from build123d import *
from build123d.topology import SkipClean

# Parameters (mm, degrees)
SKETCH7_W           = 80
SKETCH7_H           = 28
EXTRUDE2_DEPTH      = 4
SKETCH8_W           = 28
SKETCH8_H           = 20
EXTRUDE3_DEPTH      = 9.5
EXTRUDE6_DEPTH      = 28
SKETCH15_R          = 7.5
EXTRUDE7_DEPTH      = 25
SKETCH16_W          = 3
SKETCH16_H          = 3
SKETCH8_4_W         = 28
SKETCH8_4_H         = 20
EXTRUDE8_DEPTH      = 9.5
EXTRUDE9_DEPTH      = 28
SKETCH19_R          = 7.5
EXTRUDE10_DEPTH     = 25
SKETCH20_W          = 3
SKETCH20_H          = 3
FILLET1_R           = 2.5
EXTRUDE11_DEPTH     = 16
SKETCH23_R          = 4
EXTRUDE12_DEPTH     = 40
SKETCH25_W          = 28
SKETCH25_H          = 5
EXTRUDE13_DEPTH     = 12
EXTRUDE14_REACH     = 90.69
FILLET2_R           = 2.5
FILLET9_R           = 2
FILLET10_R          = 2
FILLET11_R          = 2
SKETCH27_W          = 28
SKETCH27_H          = 5
EXTRUDE15_DEPTH     = 12
EXTRUDE16_REACH     = 90.69
FILLET12_R          = 2
FILLET13_R          = 2
FILLET14_R          = 2
FILLET15_R          = 2
SKETCH30_W          = 3
SKETCH30_H          = 3
EXTRUDE17_DEPTH     = 12
SKETCH31_W          = 3
SKETCH31_H          = 3
EXTRUDE18_DEPTH     = 12
FILLET16_R          = 2
EXTRUDE19_OUTLINE_R = 1.5
EXTRUDE19_DEPTH     = 4


# Read off the part's stored shape, not the designer's step: Extrude19
with BuildPart() as part:
    # Sketch7 → Extrude2 (new body)
    with BuildSketch(Plane(origin=(0, 0, 0), x_dir=(1, 0, 0), z_dir=(0, 1, 0))):
        with Locations((0, 23)):
            Rectangle(SKETCH7_W, SKETCH7_H)
    extrude(amount=EXTRUDE2_DEPTH)


with BuildPart() as body_2:
    # Sketch8 → Extrude3 (new body)
    with BuildSketch(Plane(origin=(0, 4, 0), x_dir=(1, 0, 0), z_dir=(0, 1, 0))):
        with Locations((-23, 24)):
            Rectangle(SKETCH8_W, SKETCH8_H)
    extrude(amount=EXTRUDE3_DEPTH)

    # Sketch10 → Extrude6 (cut)
    with BuildSketch(Plane(origin=(-9, 0, 0), x_dir=(0, 0, -1), z_dir=(1, 0, 0))):
        with BuildLine():
            Line((31.5, 13.5), (24, 13.5))
            Line((24, 13.5), (16.5, 13.5))
            ThreePointArc((16.5, 13.5), (17.126403912, 10.499387259), (18.900980486, 8))
            Line((18.900980486, 8), (29.099019514, 8))
            ThreePointArc((29.099019514, 8), (30.873596088, 10.499387259), (31.5, 13.5))
        make_face()
    extrude(amount=-EXTRUDE6_DEPTH, mode=Mode.SUBTRACT)

    # Sketch15 → Extrude7 (cut)
    with SkipClean():  # the faces are left unmerged after this step: merging them gives an invalid solid
        with BuildSketch(Plane.ZY.offset(35.5)):
            with Locations((-24, 13.5)):
                Circle(SKETCH15_R)
        extrude(amount=-EXTRUDE7_DEPTH, mode=Mode.SUBTRACT)


with BuildPart() as cut_sweep1_tool:
    # Cut-Sweep1: sweep along a path in Sketch17
    with SkipClean():  # the faces are left unmerged after this step: merging them gives an invalid solid
        with BuildLine(Plane(origin=(-23, 0, 0), x_dir=(0, 0, -1), z_dir=(1, 0, 0))) as cut_sweep1_path:
            CenterArc((24, 13.5), 12.806248475, 0, 360)
        # Sketch16 → Cut-Sweep1 (sweep)
        with BuildSketch(Plane.XY.offset(-14)):
            with Locations((-23, 5.5)):
                Rectangle(SKETCH16_W, SKETCH16_H)
        sweep(path=cut_sweep1_path.line)


with BuildPart() as part_1:
    with SkipClean():  # the faces are left unmerged after this step: merging them gives an invalid solid
        add(part.part)

        # Cut-Sweep1: cut by cut_sweep1_tool
        add(cut_sweep1_tool.part, mode=Mode.SUBTRACT)

    # Sketch8<4> → Extrude8 (add)
    with BuildSketch(Plane(origin=(0, 4, 0), x_dir=(1, 0, 0), z_dir=(0, 1, 0))):
        with Locations((23, 24)):
            Rectangle(SKETCH8_4_W, SKETCH8_4_H)
    extrude(amount=EXTRUDE8_DEPTH)

    # Sketch18 → Extrude9 (cut)
    with BuildSketch(Plane(origin=(37, 0, 0), x_dir=(0, 0, -1), z_dir=(1, 0, 0))):
        with BuildLine():
            Line((18.900980486, 8), (29.099019514, 8))
            ThreePointArc((29.099019514, 8), (30.873596088, 10.499387259), (31.5, 13.5))
            Line((31.5, 13.5), (16.5, 13.5))
            ThreePointArc((16.5, 13.5), (17.126403912, 10.499387259), (18.900980486, 8))
        make_face()
    extrude(amount=-EXTRUDE9_DEPTH, mode=Mode.SUBTRACT)

    # Sketch19 → Extrude10 (cut)
    with BuildSketch(Plane(origin=(35.5, 0, 0), x_dir=(0, 0, -1), z_dir=(1, 0, 0))):
        with Locations((24, 13.5)):
            Circle(SKETCH19_R)
    extrude(amount=-EXTRUDE10_DEPTH, mode=Mode.SUBTRACT)

    # Cut-Sweep2: sweep along a path in Sketch21
    with BuildLine(Plane(origin=(23, 0, 0), x_dir=(0, 0, -1), z_dir=(1, 0, 0))) as cut_sweep2_path:
        CenterArc((24, 13.5), 12.806248475, 0, 360)
    # Sketch20 → Cut-Sweep2 (sweep, cut)
    with BuildSketch(Plane.XY.offset(-14)):
        with Locations((23, 5.5)):
            Rectangle(SKETCH20_W, SKETCH20_H)
    sweep(path=cut_sweep2_path.line, mode=Mode.SUBTRACT)

    # Fillet1
    fillet1_edges = [part_1.edges().sort_by_distance(p)[0] for p in [
        (-40, 2, -37),
        (40, 2, -37),
    ]]
    fillet(fillet1_edges, radius=FILLET1_R)

    # Sketch22 → Extrude11 (add)
    with BuildSketch(Plane(origin=(0, 0, 0), x_dir=(1, 0, 0), z_dir=(0, 1, 0))):
        Polygon((11.215030697, -11.093941854), (16, -41), (32, -41), (40, 9), (-40, 9), (-36.784969303, -11.093941854), align=None)
        Polygon((3.73640444, 4), (5.351435136, -6.093941854), (-11.084969303, -6.093941854), (-12.7, 4), align=None, mode=Mode.SUBTRACT)
        Polygon((-16.084969303, -6.093941854), (-32.521373743, -6.093941854), (-34.13640444, 4), (-17.7, 4), align=None, mode=Mode.SUBTRACT)
    extrude(amount=EXTRUDE11_DEPTH)

    # Sketch23 → Extrude12 (cut)
    with BuildSketch(Plane.XY.offset(41)):
        with Locations((24, 8)):
            Circle(SKETCH23_R)
    extrude(amount=-EXTRUDE12_DEPTH, mode=Mode.SUBTRACT)



with BuildPart() as body_2_1:
    with SkipClean():  # the faces are left unmerged after this step: merging them gives an invalid solid
        add(body_2.part)

        # Cut-Sweep1: cut by cut_sweep1_tool
        add(cut_sweep1_tool.part, mode=Mode.SUBTRACT)


with BuildPart() as part_2:
    with SkipClean():  # the faces are left unmerged after this step: merging them gives an invalid solid
        add(part_1.part)

        add(body_2_1.part)  # Extrude13 merges body 2
        # Sketch25 → Extrude13 (add)
        with BuildSketch(Plane(origin=(0, 4, 0), x_dir=(-1, 0, 0), z_dir=(0, 1, 0))):
            with Locations((23, -11.5)):
                Rectangle(SKETCH25_W, SKETCH25_H)
        extrude(amount=EXTRUDE13_DEPTH)

    # Sketch26 → Extrude14 (cut, up to next)
    with BuildSketch(Plane.ZY.offset(37), mode=Mode.PRIVATE) as extrude14_sk1:
        Polygon((-14, 13.5), (-9, 16), (-14, 16), align=None)
    extrude14_tool1 = extrude(extrude14_sk1.sketch, amount=-EXTRUDE14_REACH, mode=Mode.PRIVATE) & part_2.part
    add(extrude14_tool1.solids().sort_by_distance((-37, 15.166667, -12.333333))[0], mode=Mode.SUBTRACT)

    # Fillet2
    fillet2_edges = [part_2.edges().sort_by_distance(p)[0] for p in [
        (-36.784969303, 8, 11.093941854),
    ]]
    fillet(fillet2_edges, radius=FILLET2_R)

    # Fillet9
    fillet9_edges = [part_2.edges().sort_by_distance(p)[0] for p in [
        (-40, 10, -9),
    ]]
    fillet(fillet9_edges, radius=FILLET9_R)

    # Fillet10
    # the kernel refuses this fillet: 2 mm, written as the material it adds along each edge
    with BuildSketch(Plane(origin=(-37, 4, -9), x_dir=(0, 0, -1), z_dir=(0, 1, 0))) as fillet10_piece_1_section:
        with BuildLine():
            CenterArc((1.766934561, 2), FILLET10_R, 199.655233066, 70.344766934)
            Line((-0.11653272, 1.327280888), (-0.304879448, 1.260008977))
            ThreePointArc((-0.304879448, 1.260008977), (-0.2, 0.654561776), (-0.2, 0))
            Line((-0.2, 0), (0, -0.2))
            Line((0, -0.2), (1.766934561, -0.2))
            Line((1.766934561, -0.2), (1.766934561, 0))
        make_face()
    fillet10_piece_1 = extrude(amount=12, mode=Mode.PRIVATE)
    fillet10_piece_1 = split(fillet10_piece_1, bisect_by=Plane(origin=(-37.361885023, 14.554978546, -11.890042908), z_dir=(0, -0.8944271909999159, 0.44721359549995804)), keep=Keep.TOP, mode=Mode.PRIVATE)
    add(fillet10_piece_1)

    # Fillet11
    # the kernel refuses this fillet: 2 mm, written as the material it adds along each edge
    with BuildSketch(Plane(origin=(-9, 4, -9), x_dir=(1, 0, 0), z_dir=(0, 1, 0))) as fillet11_piece_1_section:
        with BuildLine():
            CenterArc((FILLET11_R, FILLET11_R), FILLET11_R, 180, 90)
            Line((0, FILLET11_R), (0, 0))
            Line((0, 0), (FILLET11_R, 0))
        make_face()
    fillet11_piece_1 = extrude(amount=17, mode=Mode.PRIVATE)
    fillet11_piece_1 = split(fillet11_piece_1, bisect_by=Plane(origin=(-8.54975152, 14.60165577, -11.796688461), z_dir=(0, -0.894427190999916, 0.447213595499958)), keep=Keep.TOP, mode=Mode.PRIVATE)
    add(fillet11_piece_1)

    # Sketch27 → Extrude15 (add)
    with BuildSketch(Plane(origin=(0, 4, 0), x_dir=(-1, 0, 0), z_dir=(0, 1, 0))):
        with Locations((-23, -11.5)):
            Rectangle(SKETCH27_W, SKETCH27_H)
    extrude(amount=EXTRUDE15_DEPTH)

    # Sketch28 → Extrude16 (cut, up to next)
    with BuildSketch(Plane(origin=(37, 0, 0), x_dir=(0, 0, -1), z_dir=(1, 0, 0)), mode=Mode.PRIVATE) as extrude16_sk1:
        Polygon((14, 13.5), (9, 16), (14, 16), align=None)
    extrude16_tool1 = extrude(extrude16_sk1.sketch, amount=-EXTRUDE16_REACH, mode=Mode.PRIVATE) & part_2.part
    add(extrude16_tool1.solids().sort_by_distance((37, 15.166667, -12.333333))[0], mode=Mode.SUBTRACT)

    # Fillet12
    fillet12_edges = [part_2.edges().sort_by_distance(p)[0] for p in [
        (40, 10, -9),
    ]]
    fillet(fillet12_edges, radius=FILLET12_R)

    # Fillet13
    # the kernel refuses this fillet: 2 mm, written as the material it adds along each edge
    with BuildSketch(Plane(origin=(37, -0.417336402, -9), x_dir=(0.9961678888786428, 0, 0.08746163254289291), z_dir=(0, 1, 0))) as fillet13_piece_1_section:
        with BuildLine():
            CenterArc((1.837796796, 1.935086736), FILLET13_R, 185.017593378, 70.344766934)
            Line((-0.154538981, 1.760163471), (-0.353772559, 1.742671145))
            Line((-0.353772559, 1.742671145), (-0.199233578, -0.017492327))
            Line((-0.199233578, -0.017492327), (0.017492327, -0.199233578))
            ThreePointArc((0.017492327, -0.199233578), (0.669545749, -0.141984536), (1.281845737, -0.193508674))
            Line((1.281845737, -0.193508674), (1.332386742, 0))
        make_face()
    fillet13_piece_1 = extrude(amount=16.417336402, mode=Mode.PRIVATE)
    fillet13_piece_1 = split(fillet13_piece_1, bisect_by=Plane(origin=(37.361885023, 14.554978546, -11.890042908), z_dir=(0, -0.8944271909999157, 0.4472135954999582)), keep=Keep.TOP, mode=Mode.PRIVATE)
    fillet13_piece_1 = split(fillet13_piece_1, bisect_by=Plane(origin=(37.361885023, 0, -9.612553635), z_dir=(0, 1, 0)), keep=Keep.TOP, mode=Mode.PRIVATE)
    add(fillet13_piece_1)

    # Fillet14
    # the kernel refuses this fillet: 2 mm, written as the material it adds along each edge
    with BuildSketch(Plane(origin=(9, 4, -9), x_dir=(0, 0, -1), z_dir=(0, 1, 0))) as fillet14_piece_1_section:
        with BuildLine():
            CenterArc((FILLET14_R, FILLET14_R), FILLET14_R, 180, 90)
            Line((0, FILLET14_R), (0, 0))
            Line((0, 0), (FILLET14_R, 0))
        make_face()
    fillet14_piece_1 = extrude(amount=17, mode=Mode.PRIVATE)
    fillet14_piece_1 = split(fillet14_piece_1, bisect_by=Plane(origin=(8.54975152, 14.60165577, -11.796688461), z_dir=(0, -0.894427190999916, 0.447213595499958)), keep=Keep.TOP, mode=Mode.PRIVATE)
    add(fillet14_piece_1)

    # Fillet15
    fillet15_edges = [part_2.edges().sort_by_distance(p)[0] for p in [
        (-12.7, 8, -4),
        (-11.084969303, 8, 6.093941854),
        (5.351435136, 8, 6.093941854),
        (3.73640444, 8, -4),
        (-17.7, 8, -4),
        (-34.13640444, 8, -4),
        (-32.521373743, 8, 6.093941854),
        (-16.084969303, 8, 6.093941854),
    ]]
    fillet(fillet15_edges, radius=FILLET15_R)

    # Sketch30 → Extrude17 (cut)
    with BuildSketch(Plane(origin=(0, 16, 0), x_dir=(-1, 0, 0), z_dir=(0, 1, 0))):
        with Locations((-23, -12.5)):
            Rectangle(SKETCH30_W, SKETCH30_H)
    extrude(amount=-EXTRUDE17_DEPTH, mode=Mode.SUBTRACT)

    # Sketch31 → Extrude18 (cut)
    with BuildSketch(Plane(origin=(0, 16, 0), x_dir=(-1, 0, 0), z_dir=(0, 1, 0))):
        with Locations((23, -12.5)):
            Rectangle(SKETCH31_W, SKETCH31_H)
    extrude(amount=-EXTRUDE18_DEPTH, mode=Mode.SUBTRACT)

    # Fillet16
    fillet16_edges = [part_2.edges().sort_by_distance(p)[0] for p in [
        (11.215030697, 8, 11.093941854),
    ]]
    fillet(fillet16_edges, radius=FILLET16_R)

    # Extrude19 outline → Extrude19 (cut)
    with BuildSketch(Plane(origin=(0, 0, 0), x_dir=(1, 0, 0), z_dir=(0, 1, 0))):
        with Locations((0, 22)):
            Circle(EXTRUDE19_OUTLINE_R)
        with Locations((0, 13.5)):
            Circle(EXTRUDE19_OUTLINE_R)
    extrude(amount=EXTRUDE19_DEPTH, mode=Mode.SUBTRACT)


solid = part_2.part
CAD build for the part. Positions are in the model's coordinates, mm. A direction names the side the tool comes from. Round coordinates to 2 decimals unless told otherwise and drop trailing zeros. Write each loop counter-clockwise with the first axis right and the second up, starting at its lowest first coordinate (ties: lowest second). Pieces come first, ordered by that corner, then holes. Notation, with made-up numbers: M -37,55.25 L -2,55.25 A16 cw -2,86.25 Z; hole C 23,59.25 d5. An arc over 180 degrees is marked long. Use a Markdown table: item, result. Add a question column.
1. Slice it at B-B on z = 2. Give the cut face in (x, y).
2. Pull direction Z, two halves, no side cores. Call faces 1 (the face through (-39.287, 2.028, -36.248)), 2 (the face through (36, 8, 16)), 3 (the face through (0, 4, -26)), 4 (the face through (-33.297, 8.112, -3.316)): released by +Z, released by -Z, zero draft, split by the parting line, or undercut.
3. Slice it at D-D on y = 10.5. Give the number of separate pieces and of enclosed holes in the cut face, then the cut area to 3 significant figures.
4. Flat gauge pins, fed straight in: P1, Ø2, axis at x = -22, z = -14.5, coming from the +Y side; P2, Ø0.9, axis at x = -22.5, y = 10, coming from the +Z side; P3, Ø0.9, axis at x = -23.5, y = 7.5, coming from the -Z side. Where does each tip first touch, or does it go through?
5. Slice it at C-C on z = 19. Give the cut face in (x, y), then the cut area to 3 significant figures.
6. Slice it at A-A on x = 0. Give the cut face in (y, z).
7. 3-axis set-ups, long thin cutter, end or side, ignore diameter. For faces 5 (the face through (22.979, 1.574, -23.834)), 6 (the face through (-11.835, 7.888, 1.406)), 7 (the face through (23, 9, -34)), 8 (the face through (-23, 10, -11)), 9 (the face through (-8.43, 9.92, -9.6)): which of +Z, -Z, +X, -X, +Y, -Y reach the whole face in a straight line?
8. Drill centre lines: probe 1 along Z at (x, y) = (0, 2.25); probe 2 along X at (y, z) = (1.4, -22); probe 3 along X at (y, z) = (6.5, -13). Where is each one in solid material? Low to high.
Reply:
| question | item | result |
|---|---|---|
| 1 | outline | M -38.24,0 L -33.18,0 L -33.18,16 L -38.24,16 Z; M -16.74,0 L -11.74,0 L -11.74,16 L -16.74,16 Z; M 4.7,0 L 38.24,0 L 38.24,16 L 4.7,16 Z; hole C 24,8 d8 |
| 2 | face 1 | released by -Z |
| 2 | face 2 | released by +Z |
| 2 | face 3 | zero draft |
| 2 | face 4 | undercut |
| 3 | separate pieces | 3 |
| 3 | enclosed holes | 4 |
| 3 | area | 2,200 mm^2 |
| 4 | P1 | stops at y = 13.68 |
| 4 | P2 | stops at z = 11.09 |
| 4 | P3 | stops at z = -34 |
| 5 | outline | M 12.48,0 L 35.52,0 L 35.52,16 L 12.48,16 Z; hole C 24,8 d8 |
| 5 | area | 318 mm^2 |
| 6 | outline | M 0,-37 L 4,-37 L 4,-23.5 L 0,-23.5 Z; M 0,-20.5 L 4,-20.5 L 4,-15 L 0,-15 Z; M 0,-12 L 4,-12 L 4,-9 L 16,-9 L 16,-4 L 0,-4 Z; M 0,6.09 L 16,6.09 L 16,11.09 L 0,11.09 Z |
| 7 | face 5 | none |
| 7 | face 6 | +Y, -Y |
| 7 | face 7 | -Z, +X, -X, +Y |
| 7 | face 8 | +Y |
| 7 | face 9 | -Z, +Y |
| 8 | probe 1 | z = -37 to -23.5, -20.5 to -15, -12 to -4, 6.09 to 11.09 |
| 8 | probe 2 | x = -40 to -24.5, -21.5 to -1.5, 1.5 to 21.5, 24.5 to 40 |
| 8 | probe 3 | x = -37 to -24.5, -21.5 to -9, 9 to 21.5, 24.5 to 37 |
